Geometry check sheet. Reference: drawing and pictorial views, mm from the part's lowest x, y, z. A direction names the side the tool comes from. Coordinates: 2 decimals unless noted, no trailing zeros. Loops run counter-clockwise (first coordinate to the right, second up) from the corner with the lowest first, then second, coordinate; pieces in that order, holes last.
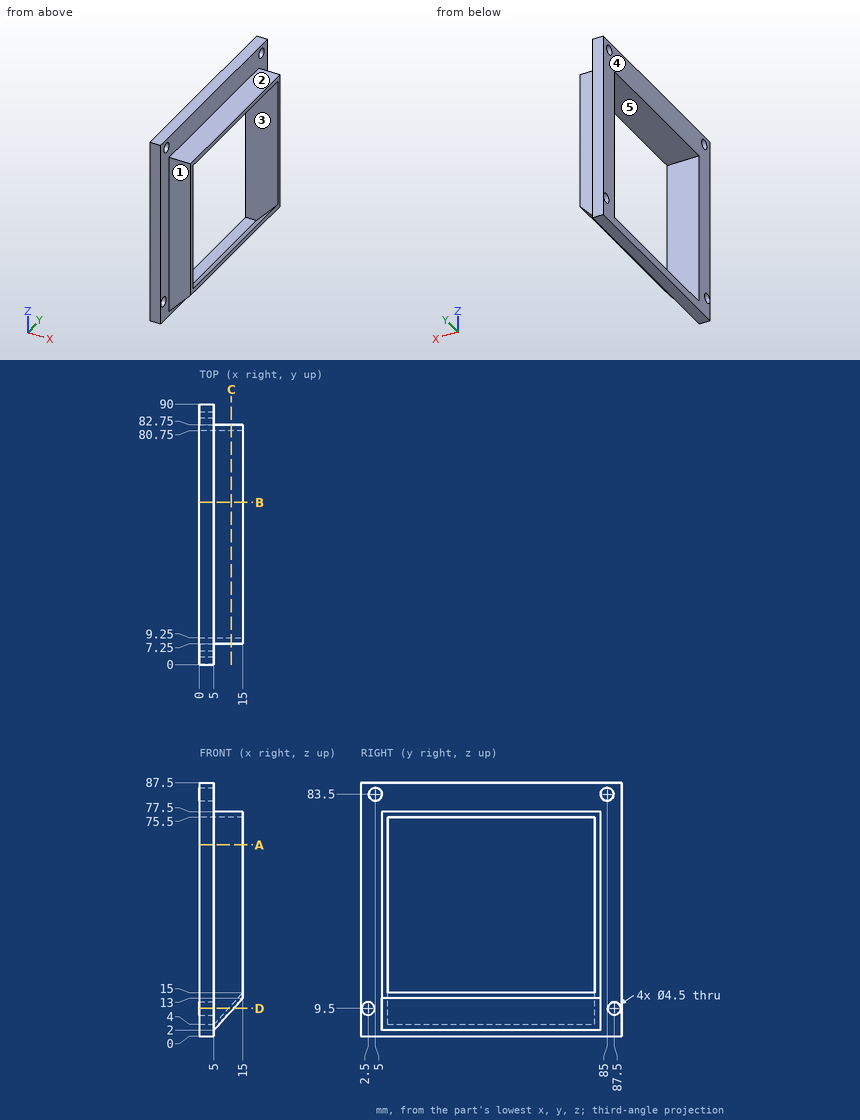
1) Material ranges on probe 1 along Y at (x, z) = (3.4, 9.5); probe 2 along Y at (x, z) = (2.35, 83.5); probe 3 along Y at (x, z) = (9.25, 74), recorded low to high.
Data:
probe 1: y = 0 to 0.25, 4.75 to 9.25, 80.75 to 85.25, 89.75 to 90
probe 2: y = 0 to 2.75, 7.25 to 82.75, 87.25 to 90
probe 3: y = 7.25 to 9.25, 80.75 to 82.75
2) Section check A-A on z = 66. Record the cut outline in (x, y), and give its area (4 significant figures).
Data:
outline: (0, 0) - (5, 0) - (5, 7.25) - (15, 7.25) - (15, 9.25) - (0, 9.25) - close; (0, 80.75) - (15, 80.75) - (15, 82.75) - (5, 82.75) - (5, 90) - (0, 90) - close
area: 132.5 mm2
3) Depth check by flat-ended pin: pin 1 (2 mm diameter, centred on x = 11.5, y = 39.5, fed in from -Z); pin 2 (5 mm diameter, centred on x = 12, y = 26.5, fed in from +Z). Enter the tip coordinate at first touch or a pass-through.
Data:
pin 1: stops at z = 8.05
pin 2: stops at z = 77.5
4) Section check D-D on z = 9.5. Record the cut outline in (x, y), and give its area (3 significant figures).
Data:
outline: (0, 0) - (5, 0) - (5, 0.25) - (0, 0.25) - close; (0, 4.75) - (5, 4.75) - (5, 7.25) - (11.82, 7.25) - (11.82, 82.75) - (5, 82.75) - (5, 85.25) - (0, 85.25) - (0, 80.75) - (10, 80.75) - (10, 9.25) - (0, 9.25) - close; (0, 89.75) - (5, 89.75) - (5, 90) - (0, 90) - close
area: 205 mm2
5) Access from +Z, -Z, +X, -X, +Y, -Y to the whole of each face (thin tool, end or side, straight path). Record for the marked faces 4 and 5.
Data:
face 4: +Z, -Z, -X, +Y, -Y
face 5: +X, -X
6) Section check B-B on y = 56. Record the cut outline in (x, z), and give its area (3 significant figures).
Data:
outline: (0, 0) - (5, 0) - (5, 2) - (15, 13) - (15, 15) - (5, 4) - (0, 4) - close; (0, 75.5) - (15, 75.5) - (15, 77.5) - (5, 77.5) - (5, 87.5) - (0, 87.5) - close
area: 120 mm2
7) Mould release check, pull along Z, two halves, no side actions. Record for the marked faces 1, 2 and 3: +Z half, -Z half, draft (parallel to the pull), parting line (faces both ways), or undercut.
Data:
face 1: draft
face 2: +Z half
face 3: undercut
8) Section check C-C on x = 11. Record the cut outline in (y, z).
Data:
outline: (7.25, 8.6) - (82.75, 8.6) - (82.75, 77.5) - (7.25, 77.5) - close; hole (9.25, 10.6) - (80.75, 10.6) - (80.75, 75.5) - (9.25, 75.5) - close
